Autodesk Inventor part; units mm, degrees
ref_plane "YZ Plane" through (0, 0, 0) normal (1, 0, 0) x (0, 1, 0)
ref_plane "XZ Plane" through (0, 0, 0) normal (0, 1, 0) x (-1, 0, 0)
ref_plane "XY Plane" through (0, 0, 0) normal (0, 0, 1) x (1, 0, 0)
sketch "Эскиз1" plane through (0, 0, 0) normal (0, 0, 1) x (1, 0, 0)
  circle A0 centre (0, 0) radius 132.5
  dimension "d0" = 265
extrude "Выдавливание1" add sketch "Эскиз1" along normal mid plane 6
sketch "Эскиз2" plane through (0, 0, -3) normal (0, 0, -1) x (-1, 0, 0)
  circle A0 centre (20, -124.909) radius 1.6
  circle A1 centre (-20, -124.909) radius 1.6
  point P0 (0, 0)
extrude "Выдавливание2" cut sketch "Эскиз2" against normal through all
pattern_circular "Круговой массив1" count 3 over 360 about axis through (0, 0, -10) along (0, 0, 1) of "Выдавливание2"
sketch "Эскиз3" plane through (0, 0, 3) normal (0, 0, 1) x (1, 0, 0)
  line L0 (-5, -5) -> (5, -5) construction
  line L1 (5, -5) -> (5, 5) construction
  line L2 (5, 5) -> (-5, 5) construction
  line L3 (-5, 5) -> (-5, -5) construction
  line L4 (-5, -5) -> (5, 5) construction
  line L5 (5, -5) -> (-5, 5) construction
  point P0 (0, 0)
  dimension "d8" = 10
hole "Отверстие1" at (-5, 5, 3) at (5, 5, 3) at (-5, -5, 3) at (5, -5, 3) direction (0, 0, -1) diameter 3.2 end through all
properties part number "Диск опорный"
Can you work these out from the model? Positions are in its coordinate system, mm. Coordinates: 2 decimals unless noted, no trailing zeros. Loops run counter-clockwise (first coordinate to the right, second up) from the corner with the lowest first, then second, coordinate; pieces in that order, holes last.
1) Imagine slicing it at B-B on x = 53.5. List the corners of the cut face in (y, z) for me, plus the area to 3 significant figures.
2) Imagine slicing it at A-A on z = 0.75. State how many separate pieces and enclosed holes the cut face has, plus the area to 3 significant figures.
3) For pin 1 (1.9 mm diameter, centred on x = -118.17, y = 45.13, fed in from -Z); pin 2 (1 mm diameter, centred on y = -78.5, z = 2, fed in from -X); pin 3 (1.5 mm diameter, centred on y = -75, z = -1.5, fed in from +X), each with a flat end and sliding along its axis, tell me the tip position at first contact or that it passes through.
4) I need wall thicknesses on probe 1 along Y at (x, z) = (5, -0.3); probe 2 along Y at (x, z) = (20, 0.85); probe 3 along Y at (x, z) = (102.5, -1.35). Which ranges of each line are inside material? Lowest first, please.
5) Imagine slicing it at C-C on y = -62.5. List the corners of the cut face in (x, z) for me.
Completed:
1. outline: (-121.22, -3) - (121.22, -3) - (121.22, 3) - (-121.22, 3) - close
1. area: 1,450 mm2
2. separate pieces: 1
2. enclosed holes: 10
2. area: 55,100 mm2
3. pin 1: passes through
3. pin 2: stops at x = -107.11
3. pin 3: stops at x = 109.74
4. probe 1: y = -132.41 to -6.6, -3.4 to 3.4, 6.6 to 132.41
4. probe 2: y = -130.98 to -126.51, -123.31 to 130.98
4. probe 3: y = -83.96 to 83.96
5. outline: (-116.83, -3) - (116.83, -3) - (116.83, 3) - (-116.83, 3) - close
